from build123d import *

# Parameters (mm, degrees)
ESQUISSE1_W             = 60
ESQUISSE1_H             = 42.3
ESQUISSE1_R             = 2
BOSS_EXTRU_1_DEPTH      = 10
ESQUISSE2_R             = 11
ENL_V_MAT_EXTRU_1_DEPTH = 10
CONG_1_R                = 2


with BuildPart() as part:
    # Esquisse1 → Boss.-Extru.1 (new body)
    with BuildSketch(Plane.XY):
        Rectangle(ESQUISSE1_W, ESQUISSE1_H)
        with Locations((15.5, 15.5)):
            Circle(ESQUISSE1_R, mode=Mode.SUBTRACT)
        with Locations(Location((-15.5, 15.5, 0), (0, 0, 180))):
            Circle(ESQUISSE1_R, mode=Mode.SUBTRACT)
        with Locations(Location((15.5, -15.5, 0), (0, 0, 180))):
            Circle(ESQUISSE1_R, mode=Mode.SUBTRACT)
        with Locations((-15.5, -15.5)):
            Circle(ESQUISSE1_R, mode=Mode.SUBTRACT)
        with Locations((25, 16.15)):
            Circle(ESQUISSE1_R, mode=Mode.SUBTRACT)
        with Locations(Location((-25, 16.15, 0), (0, 0, 180))):
            Circle(ESQUISSE1_R, mode=Mode.SUBTRACT)
        with Locations((-25, -16.15)):
            Circle(ESQUISSE1_R, mode=Mode.SUBTRACT)
        with Locations(Location((25, -16.15, 0), (0, 0, 180))):
            Circle(ESQUISSE1_R, mode=Mode.SUBTRACT)
    extrude(amount=BOSS_EXTRU_1_DEPTH)

    # Esquisse2 → Enlèv. mat.-Extru.1 (cut)
    with BuildSketch(Plane.XY.offset(10)):
        Circle(ESQUISSE2_R)
    extrude(amount=-ENL_V_MAT_EXTRU_1_DEPTH, mode=Mode.SUBTRACT)

    # Congé1
    cong_1_edges = [part.edges().sort_by_distance(p)[0] for p in [
        (30, -21.15, 5),
        (-30, -21.15, 5),
        (-30, 21.15, 5),
        (30, 21.15, 5),
    ]]
    fillet(cong_1_edges, radius=CONG_1_R)


solid = part.part
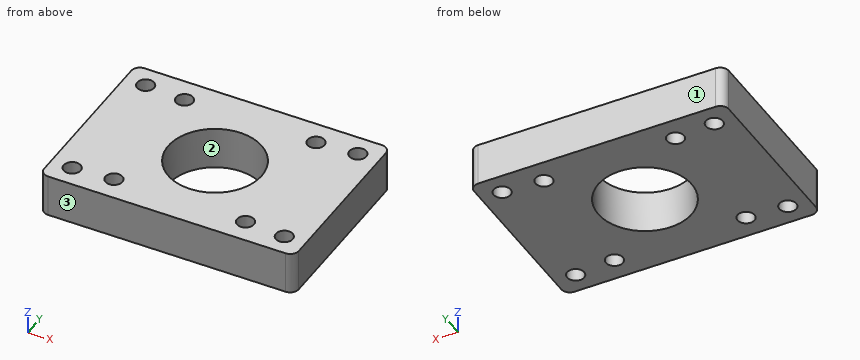
Input: part model. Units: mm. Frame: model coordinates. Face numbers are marked on the shaded views. Coordinates: 2 decimals unless noted, no trailing zeros. Loops run counter-clockwise (first coordinate to the right, second up) from the corner with the lowest first, then second, coordinate; pieces in that order, holes last.
Q1. Cut plane B-B (x = 0). Output: boundary loops of the cut face in (y, z), then the cut area to 3 significant figures.
Q2. Cut plane A-A (y = 0). Output: boundary loops of the cut face in (x, z).
Q3. Cut plane C-C (x = 15.5). Output: boundary loops of the cut face in (y, z), then the cut area to 3 significant figures.
Q4. Draft query along Y for the marked faces 1, 2 and 3. Return one class per face: +Y half, -Y half, draft (parallel to the pull), parting line (faces both ways), or undercut.
Q5. Contact query for a flat-ended pin moving along its axis: pin 1 (3.5 mm diameter, centred on x = -15.5, y = -15.5, fed in from -Z). Output: stop coordinate, or through.
Q6. Cut plane D-D (z = 3.75). Give the number of separate pieces and of enclosed holes in the cut face, then the cut area to 3 significant figures.
Q7. Material intervals for line 1 (Y direction, x = -25, z = 3.75); line 2 (Y direction, x = 15.5, z = 6.5); line 3 (X direction, y = -17, z = 2.5), sorted ascending.
Working result:
1. outline: (-21.15, 0) - (-11, 0) - (-11, 10) - (-21.15, 10) - close; (11, 0) - (21.15, 0) - (21.15, 10) - (11, 10) - close
1. area: 203 mm2
2. outline: (-30, 0) - (-11, 0) - (-11, 10) - (-30, 10) - close; (11, 0) - (30, 0) - (30, 10) - (11, 10) - close
3. outline: (-21.15, 0) - (-17.5, 0) - (-17.5, 10) - (-21.15, 10) - close; (-13.5, 0) - (13.5, 0) - (13.5, 10) - (-13.5, 10) - close; (17.5, 0) - (21.15, 0) - (21.15, 10) - (17.5, 10) - close
3. area: 343 mm2
4. face 1: +Y half
4. face 2: undercut
4. face 3: -Y half
5. pin 1: passes through
6. separate pieces: 1
6. enclosed holes: 9
6. area: 2,050 mm2
7. line 1: y = -21.15 to -18.15, -14.15 to 14.15, 18.15 to 21.15
7. line 2: y = -21.15 to -17.5, -13.5 to 13.5, 17.5 to 21.15
7. line 3: x = -30 to -26.81, -23.19 to -16.82, -14.18 to 14.18, 16.82 to 23.19, 26.81 to 30
